Input: part model. Units: mm. Frame: model coordinates. A direction names the side the tool comes from. Round coordinates to 2 decimals unless told otherwise and drop trailing zeros. Order: outer loops, then holes, each group sorted by start corner. A loop starts at its lowest first (then second) coordinate and runs counter-clockwise, first axis right, second up. Notation, with made-up numbers: (22, 13) - (31, 13) arc R13 ccw to (31, 23) - close; hole circle Ø10 at (63, 78). An arc over 180 degrees is marked (long way). One line per item, written item: value. Start each with the question number.
from build123d import *

# Parameters (mm, degrees)
SKETCH_1_R                   = 15
EXTRUDE_1_DEPTH              = 25
SKETCH_5_W                   = 20
SKETCH_5_H                   = 120
CUT_EXTRUDE_1_DEPTH          = 6
FILLET_1_R                   = 5
FILLET_2_R                   = 5
FILLET_3_R                   = 5
FILLET_4_R                   = 5
FILLET_5_R                   = 5
FILLET_6_R                   = 5
SKETCH_7_R                   = 5.5
CUT_EXTRUDE_2_DEPTH          = 270.256549022
SKETCH_8_R                   = 8.5
CUT_EXTRUDE_3_DEPTH          = 10
HOLE_WIZARD_M8_1_D           = 6.8
HOLE_WIZARD_M8_1_DEPTH       = 9.75
HOLE_WIZARD_M8_1_CBORE_D     = 8
HOLE_WIZARD_M8_1_CBORE_DEPTH = 6
HOLE_WIZARD_M8_1_TIP         = 2.042926105
HOLE_WIZARD_M8_2_D           = 6.8
HOLE_WIZARD_M8_2_DEPTH       = 9.75
HOLE_WIZARD_M8_2_CBORE_D     = 8
HOLE_WIZARD_M8_2_CBORE_DEPTH = 6
HOLE_WIZARD_M8_2_TIP         = 2.042926105
FILLET_7_R                   = 2
CHAMFER_1_SIZE               = 2
CHAMFER_2_SIZE               = 1
CHAMFER_3_SIZE               = 1
HOLE_WIZARD_M3_1_D           = 2.5
HOLE_WIZARD_M3_1_DEPTH       = 7.5
HOLE_WIZARD_M3_1_CBORE_D     = 3
HOLE_WIZARD_M3_1_CBORE_DEPTH = 6
HOLE_WIZARD_M3_1_TIP         = 0.751075774
SKETCH_15_R                  = 1.05
CUT_EXTRUDE_4_DEPTH          = 10


with BuildPart() as part:
    # 草图1 → 拉伸1 (new body)
    with BuildSketch(Plane.XY):
        Polygon((-107.694965591, 220.629249387), (-137.694965591, 168.66772516), (-22.694965591, -30.518117711), (37.305034409, -30.518117711), (152.305034409, 168.66772516), (122.305034409, 220.629249387), align=None)
        with Locations((7.305034409, 119.592952279)):
            Circle(SKETCH_1_R, mode=Mode.SUBTRACT)
    extrude(amount=EXTRUDE_1_DEPTH)

    # 草图5 → 切除-拉伸1 (cut)
    with BuildSketch(Plane(origin=(0, 0, 0), x_dir=(-1, 0, 0), z_dir=(0, 0, -1))):
        Polygon((26.762298194, 150.808741311), (130.669741536, 210.799731695), (125.132108132, 230.696588327), (16.762298194, 168.129249387), align=None)
        Polygon((-170.362424446, 179.093164159), (-61.372367011, 116.16772516), (-51.372367011, 133.488233235), (-160.362424446, 196.413672234), align=None)
        with Locations((12.694965591, 14.481882289)):
            Rectangle(SKETCH_5_W, SKETCH_5_H)
    extrude(amount=-CUT_EXTRUDE_1_DEPTH, mode=Mode.SUBTRACT)

    # 圆角1
    fillet_1_edges = [part.edges().sort_by_distance(p)[0] for p in [
        (-16.762298194, 168.129249387, 3),
    ]]
    fillet(fillet_1_edges, radius=FILLET_1_R)

    # 圆角2
    fillet_2_edges = [part.edges().sort_by_distance(p)[0] for p in [
        (-26.762298194, 150.808741311, 3),
    ]]
    fillet(fillet_2_edges, radius=FILLET_2_R)

    # 圆角3
    fillet_3_edges = [part.edges().sort_by_distance(p)[0] for p in [
        (61.372367011, 116.16772516, 3),
    ]]
    fillet(fillet_3_edges, radius=FILLET_3_R)

    # 圆角4
    fillet_4_edges = [part.edges().sort_by_distance(p)[0] for p in [
        (51.372367011, 133.488233235, 3),
    ]]
    fillet(fillet_4_edges, radius=FILLET_4_R)

    # 圆角5
    fillet_5_edges = [part.edges().sort_by_distance(p)[0] for p in [
        (-22.694965591, 74.481882289, 3),
    ]]
    fillet(fillet_5_edges, radius=FILLET_5_R)

    # 圆角6
    fillet_6_edges = [part.edges().sort_by_distance(p)[0] for p in [
        (-2.694965591, 74.481882289, 3),
    ]]
    fillet(fillet_6_edges, radius=FILLET_6_R)

    # 草图7 → 切除-拉伸2 (cut, through all)
    with BuildSketch(Plane(origin=(0, 0, 0), x_dir=(-1, 0, 0), z_dir=(0, 0, -1))):
        with Locations((104.034711553, 206.968995349)):
            Circle(SKETCH_7_R)
        with Locations((34.752679251, 166.968995349)):
            Circle(SKETCH_7_R)
        with Locations((-138.644780371, 172.327979198)):
            Circle(SKETCH_7_R)
        with Locations((-69.362748068, 132.327979198)):
            Circle(SKETCH_7_R)
        with Locations((12.694965591, 59.481882289)):
            Circle(SKETCH_7_R)
        with Locations((12.694965591, -20.518117711)):
            Circle(SKETCH_7_R)
    extrude(amount=-CUT_EXTRUDE_2_DEPTH, mode=Mode.SUBTRACT)

    # 草图8 → 切除-拉伸3 (cut)
    with BuildSketch(Plane.XY.offset(25)):
        with Locations((-12.694965591, 59.481882289)):
            Circle(SKETCH_8_R)
        with Locations((-12.694965591, -20.518117711)):
            Circle(SKETCH_8_R)
        with Locations((69.362748068, 132.327979198)):
            Circle(SKETCH_8_R)
        with Locations((138.644780371, 172.327979198)):
            Circle(SKETCH_8_R)
        with Locations((-34.752679251, 166.968995349)):
            Circle(SKETCH_8_R)
        with Locations((-104.034711553, 206.968995349)):
            Circle(SKETCH_8_R)
    extrude(amount=-CUT_EXTRUDE_3_DEPTH, mode=Mode.SUBTRACT)

    # M8 螺纹孔1
    with Locations(Plane(origin=(0, 0, 0), x_dir=(-1, 0, 0), z_dir=(0, 0, -1))):
        with Locations((-42.305034409, 119.592952279), (-7.305034409, 154.592952279), (27.694965591, 119.592952279), (-7.305034409, 84.592952279)):
            CounterBoreHole(HOLE_WIZARD_M8_1_D / 2, HOLE_WIZARD_M8_1_CBORE_D / 2, HOLE_WIZARD_M8_1_CBORE_DEPTH, depth=HOLE_WIZARD_M8_1_DEPTH)
            with Locations((0, 0, -(HOLE_WIZARD_M8_1_DEPTH + HOLE_WIZARD_M8_1_TIP / 2))):  # 118° drill point
                Cone(0, HOLE_WIZARD_M8_1_D / 2, HOLE_WIZARD_M8_1_TIP, mode=Mode.SUBTRACT)

    # M8 螺纹孔2
    with Locations(Plane.XY.offset(25)):
        with Locations((32.05377175, 94.844214937), (32.05377175, 144.34168962), (-17.410599553, 144.374748781), (-17.410599553, 94.811155776)):
            CounterBoreHole(HOLE_WIZARD_M8_2_D / 2, HOLE_WIZARD_M8_2_CBORE_D / 2, HOLE_WIZARD_M8_2_CBORE_DEPTH, depth=HOLE_WIZARD_M8_2_DEPTH)
            with Locations((0, 0, -(HOLE_WIZARD_M8_2_DEPTH + HOLE_WIZARD_M8_2_TIP / 2))):  # 118° drill point
                Cone(0, HOLE_WIZARD_M8_2_D / 2, HOLE_WIZARD_M8_2_TIP, mode=Mode.SUBTRACT)

    # 圆角7
    fillet_7_edges = [part.edges().sort_by_distance(p)[0] for p in [
        (147.305034409, 177.327979198, 6),
        (-112.694965591, 211.968995349, 6),
        (-12.694965591, -30.518117711, 6),
    ]]
    fillet(fillet_7_edges, radius=FILLET_7_R)

    # 倒角1
    chamfer_1_edges = [part.edges().sort_by_distance(p)[0] for p in [
        (-7.694965591, 119.592952279, 0),
    ]]
    chamfer(chamfer_1_edges, length=CHAMFER_1_SIZE)

    # 倒角2
    chamfer_2_edges = [part.edges().sort_by_distance(p)[0] for p in [
        (-112.534711553, 206.968995349, 25),
    ]]
    chamfer(chamfer_2_edges, length=CHAMFER_2_SIZE)

    # 倒角3
    chamfer_3_edges = [part.edges().sort_by_distance(p)[0] for p in [
        (-21.194965591, 59.481882289, 25),
        (-21.194965591, -20.518117711, 25),
        (60.862748068, 132.327979198, 25),
        (130.144780371, 172.327979198, 25),
        (-7.694965591, 119.592952279, 25),
        (-43.252679251, 166.968995349, 25),
    ]]
    chamfer(chamfer_3_edges, length=CHAMFER_3_SIZE)

    # M3 螺纹孔1
    with Locations(Plane(origin=(0.805034409, 83.992952279, 25), x_dir=(1, 0, 0), z_dir=(0, 0, 1))):
        with Locations((0, 0)):
            CounterBoreHole(HOLE_WIZARD_M3_1_D / 2, HOLE_WIZARD_M3_1_CBORE_D / 2, HOLE_WIZARD_M3_1_CBORE_DEPTH, depth=HOLE_WIZARD_M3_1_DEPTH)
            with Locations((0, 0, -(HOLE_WIZARD_M3_1_DEPTH + HOLE_WIZARD_M3_1_TIP / 2))):  # 118° drill point
                Cone(0, HOLE_WIZARD_M3_1_D / 2, HOLE_WIZARD_M3_1_TIP, mode=Mode.SUBTRACT)

    # 草图15 → 切除-拉伸4 (cut)
    with BuildSketch(Plane.XY.offset(25)):
        with Locations((7.305034409, 99.592952279)):
            Circle(SKETCH_15_R)
    extrude(amount=-CUT_EXTRUDE_4_DEPTH, mode=Mode.SUBTRACT)


solid = part.part
1. Section A-A (x = -50). Return the cut outline in (y, z).
2. Pull-direction query (X, two-part tool) for faces 1 (the face through (-81, 70.47, 12.32)), 2 (the face through (-22.695, 19, 3)), 3 (the face through (94, 67.68, 12.32)); classes: released by +X, released by -X, zero draft, split by the parting line, or undercut.
3. Section B-B (y = 13). Return the cut outline in (x, z).
4. Set-up query: faces 4 (the face through (10, 87, 6)), 5 (the face through (-13, 24, 6)), 6 (the face through (31.53, 98.81, 22.04)), 7 (the face through (-122.485, 195.012, 12.325)). Return all of +Z, -Z, +X, -X, +Y, -Y with unobstructed straight access to the full face (end or side cutting, diameter ignored); none if empty.
5. Pin query (flat end, axial travel): pin 1 (3 mm diameter, centred on y = 152.5, z = 12, fed in from -X); pin 2 (2 mm diameter, centred on x = 50.5, z = 8, fed in from -Y); pin 3 (7 mm diameter, centred on x = 32.05, y = 94.84, fed in from +Z); pin 4 (9 mm diameter, centred on x = -104.03, y = 206.97, fed in from +Z). Return the tip coordinate at first contact, or that it passes through.
6. Line query: line 1 (Y direction, x = -91, z = 4); line 2 (X direction, y = 63, z = 22.5); line 3 (X direction, y = 139, z = 22.25). Output: solid intervals per line, ascending. Write a range as from..to.
Solved:
1. outline: (16.78, 0) - (164.23, 0) - (164.23, 6) - (187.32, 6) - (187.32, 0) - (220.63, 0) - (220.63, 25) - (16.78, 25) - close
2. face 1: released by -X
2. face 2: undercut
2. face 3: released by +X
3. outline: (-47.82, 0) - (-22.69, 0) - (-22.69, 6) - (-2.69, 6) - (-2.69, 0) - (62.43, 0) - (62.43, 25) - (-47.82, 25) - close
4. face 4: -Z
4. face 5: -Z, -Y
4. face 6: +Z
4. face 7: +Z, -Z, -X, +Y
5. pin 1: stops at x = -129.23
5. pin 2: stops at y = -9.4
5. pin 3: stops at z = 19
5. pin 4: passes through
6. line 1: y = 87.79..187.9, 210.99..220.63
6. line 2: x = -76.69..-20.43, -4.96..91.3
6. line 3: x = -120.57..64.1, 74.63..135.18
